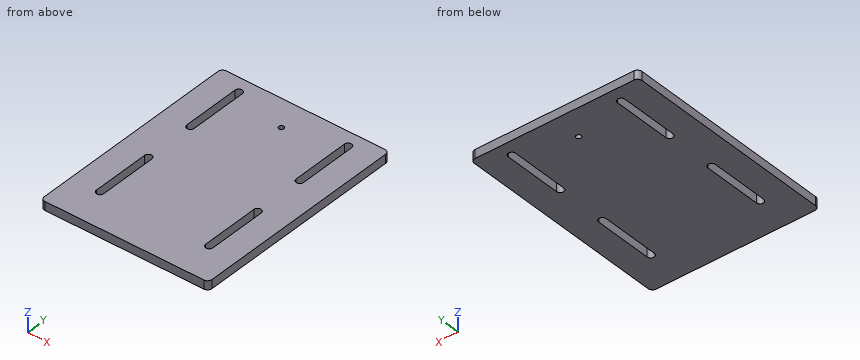
```python
from build123d import *

# Parameters (mm, degrees)
F1_DEPTH = 6
F3_DEPTH = 6
F4_R     = 1.75
F5_DEPTH = 6


with BuildPart() as f1:
    # F0 (on Top) → F1 (new body)
    with BuildSketch(Plane.XY):
        with BuildLine():
            Line((-54.5, -75), (54.5, -75))
            ThreePointArc((54.5, -75), (56.62132, -74.12132), (57.5, -72))
            Line((57.5, -72), (57.5, 72))
            ThreePointArc((57.5, 72), (56.62132, 74.12132), (54.5, 75))
            Line((54.5, 75), (-54.5, 75))
            ThreePointArc((-54.5, 75), (-56.62132, 74.12132), (-57.5, 72))
            Line((-57.5, 72), (-57.5, -72))
            ThreePointArc((-57.5, -72), (-56.62132, -74.12132), (-54.5, -75))
        make_face()
    extrude(amount=F1_DEPTH)

    # F2 (on face) → F3 (cut, through all)
    with BuildSketch(Plane.XY.offset(6)):
        with BuildLine():
            ThreePointArc((-35, 65), (-37.5, 67.5), (-40, 65))
            Line((-40, 65), (-40, 25))
            ThreePointArc((-40, 25), (-37.5, 22.5), (-35, 25))
            Line((-35, 25), (-35, 65))
        make_face()
        with BuildLine():
            ThreePointArc((40, 65), (37.5, 67.5), (35, 65))
            Line((35, 65), (35, 25))
            ThreePointArc((35, 25), (37.5, 22.5), (40, 25))
            Line((40, 25), (40, 65))
        make_face()
        with BuildLine():
            ThreePointArc((40, -10), (37.5, -7.5), (35, -10))
            Line((35, -10), (35, -50))
            ThreePointArc((35, -50), (37.5, -52.5), (40, -50))
            Line((40, -50), (40, -10))
        make_face()
        with BuildLine():
            ThreePointArc((-35, -10), (-37.5, -7.5), (-40, -10))
            Line((-40, -10), (-40, -50))
            ThreePointArc((-40, -50), (-37.5, -52.5), (-35, -50))
            Line((-35, -50), (-35, -10))
        make_face()
    extrude(amount=-F3_DEPTH, mode=Mode.SUBTRACT)

    # F4 (on face) → F5 (cut, through all)
    with BuildSketch(Plane.XY.offset(6)):
        with Locations((0, 55)):
            Circle(F4_R)
    extrude(amount=-F5_DEPTH, mode=Mode.SUBTRACT)


solid = f1.part
```
Geometry: final body of the model. Coordinates: model frame, mm. Give positions to 0.01 mm unless a question says otherwise; leave off trailing zeros. Loops run counter-clockwise (first coordinate to the right, second up) from the corner with the lowest first, then second, coordinate; pieces in that order, holes last. Notation, with made-up numbers: (14, 62) -> (18, 62) arc R13 ccw to (18, 83) -> close; hole circle Ø11 at (85, -22). An arc over 180 degrees is marked (long way). Use CSV: the item, a comma, the result in double quotes.
(1) Ray query, line 1 along X through (y, z) = (-40.5, 3.8); line 2 along Y through (x, z) = (0, 3.75); line 3 along X through (y, z) = (54.5, 4.7). Return the intervals inside material, ascending. Write a range as [from, to].
From the geometry:
line 1,"[-57.5, -40], [-35, 35], [40, 57.5]"
line 2,"[-75, 53.25], [56.75, 75]"
line 3,"[-57.5, -40], [-35, -1.68], [1.68, 35], [40, 57.5]"
(2) First-contact query: P1, Ø6, axis at x = 3.5, y = -25.5, coming from the -Z side. Flat tip, straight axial feed; report the tip coordinate or a pass-through.
From the geometry:
P1,"z = 0"
(3) Cut plane B-B (x = 0). Output: boundary loops of the cut face in (y, z).
From the geometry:
outline,"(-75, 0) -> (53.25, 0) -> (53.25, 6) -> (-75, 6) -> close; (56.75, 0) -> (75, 0) -> (75, 6) -> (56.75, 6) -> close"
(4) Cut plane A-A (y = 55). Output: boundary loops of the cut face in (x, z).
From the geometry:
outline,"(-57.5, 0) -> (-40, 0) -> (-40, 6) -> (-57.5, 6) -> close; (-35, 0) -> (-1.75, 0) -> (-1.75, 6) -> (-35, 6) -> close; (1.75, 0) -> (35, 0) -> (35, 6) -> (1.75, 6) -> close; (40, 0) -> (57.5, 0) -> (57.5, 6) -> (40, 6) -> close"
(5) Cut plane C-C (z = 2.65). Output: boundary loops of the cut face in (x, y), plus the area to 3 significant figures.
From the geometry:
outline,"(-57.5, -72) arc R3 ccw to (-54.5, -75) -> (54.5, -75) arc R3 ccw to (57.5, -72) -> (57.5, 72) arc R3 ccw to (54.5, 75) -> (-54.5, 75) arc R3 ccw to (-57.5, 72) -> close; hole (-40, -50) arc R2.5 ccw to (-35, -50) -> (-35, -10) arc R2.5 ccw to (-40, -10) -> close; hole (-40, 25) arc R2.5 ccw to (-35, 25) -> (-35, 65) arc R2.5 ccw to (-40, 65) -> close; hole circle Ø3.5 at (0, 55); hole (35, -50) arc R2.5 ccw to (40, -50) -> (40, -10) arc R2.5 ccw to (35, -10) -> close; hole (35, 25) arc R2.5 ccw to (40, 25) -> (40, 65) arc R2.5 ccw to (35, 65) -> close"
area,"16,400 mm^2"
(6) Cut plane D-D (y = 30). Output: boundary loops of the cut face in (x, z).
From the geometry:
outline,"(-57.5, 0) -> (-40, 0) -> (-40, 6) -> (-57.5, 6) -> close; (-35, 0) -> (35, 0) -> (35, 6) -> (-35, 6) -> close; (40, 0) -> (57.5, 0) -> (57.5, 6) -> (40, 6) -> close"
